from build123d import *

# Parameters (mm, degrees)
SKETCH1_R           = 7.25
BOSS_EXTRUDE1_DEPTH = 3
SKETCH2_R           = 3.5
SKETCH2_R_2         = 2.5
BOSS_EXTRUDE2_DEPTH = 3
SKETCH3_R           = 0.75
CUT_EXTRUDE1_DEPTH  = 12.879604371
CHAMFER1_SIZE       = 0.5
SKETCH5_R           = 1.25
CUT_EXTRUDE3_DEPTH  = 12.879604371


with BuildPart() as part:
    # Sketch1 → Boss-Extrude1 (new body)
    with BuildSketch(Plane.XY):
        Circle(SKETCH1_R)
    extrude(amount=BOSS_EXTRUDE1_DEPTH)

    # Sketch2 → Boss-Extrude2 (add)
    with BuildSketch(Plane(origin=(0, 0, 0), x_dir=(-1, 0, 0), z_dir=(0, 0, -1))):
        with Locations(Location((0, 0, 0), (0, 0, 180))):
            Circle(SKETCH2_R)
        Circle(SKETCH2_R_2, mode=Mode.SUBTRACT)
    extrude(amount=BOSS_EXTRUDE2_DEPTH)

    # Sketch3 → Cut-Extrude1 (cut, through all)
    with BuildSketch(Plane.XY.offset(3)):
        with Locations((0, 5)):
            Circle(SKETCH3_R)
        with Locations((5, 0)):
            Circle(SKETCH3_R)
        with Locations((0, -5)):
            Circle(SKETCH3_R)
        with Locations((-5, 0)):
            Circle(SKETCH3_R)
    extrude(amount=-CUT_EXTRUDE1_DEPTH, mode=Mode.SUBTRACT)

    # Chamfer1
    chamfer1_edges = [part.edges().sort_by_distance(p)[0] for p in [
        (-7.25, 0, 0),
        (-7.25, 0, 3),
        (-3.5, 0, -3),
    ]]
    chamfer(chamfer1_edges, length=CHAMFER1_SIZE)

    # Sketch5 → Cut-Extrude3 (cut, through all)
    with BuildSketch(Plane.XY.offset(3)):
        Circle(SKETCH5_R)
    extrude(amount=-CUT_EXTRUDE3_DEPTH, mode=Mode.SUBTRACT)


solid = part.part
Here's how the part is built. I have some questions about the finished solid (model axes, mm). A direction names the side the tool comes from. Coordinates: 2 decimals unless noted, no trailing zeros. Order: outer loops, then holes, each group sorted by start corner. A loop starts at its lowest first (then second) coordinate and runs counter-clockwise, first axis right, second up. Notation, with made-up numbers: (19.5, 30.25) -> (26.5, 30.25) arc R16 cw to (26.5, 49.25) -> close; hole circle Ø5 at (28, 74.25). An arc over 180 degrees is marked (long way). Answer in a Markdown table with one row per item.
(1) Thinking about a two-plate mould opening in Y: for faces 1 (the face through (3.35, -6.43, 1.49)), 2 (the face through (-0.27, -1.22, 1.52)), 3 (the face through (1.4, 0.1, 3)), 4 (the face through (0.54, -2.44, -1.48)), which applies, +Y half, -Y half, draft (parallel to the pull), parting line (faces both ways), or undercut?
Answer key:
| item | result |
|---|---|
| face 1 | parting line |
| face 2 | undercut |
| face 3 | draft |
| face 4 | undercut |
(2) Will these pins go through, and if not, where does the flat tip stop? pin 1 Ø1 at (x, z) = (-6, 0) entering from -Y; pin 2 Ø4 at (x, y) = (5, -4.5) entering from -Z.
Answer key:
| item | result |
|---|---|
| pin 1 | y = -4.32 |
| pin 2 | z = 0 |
(3) I want a section at A-A on x = 0. Count the separate pieces of the cut face and the enclosed holes in it, then the cut area to 4 significant figures.
Answer key:
| item | result |
|---|---|
| separate pieces | 4 |
| enclosed holes | 0 |
| area | 32.25 mm^2 |
(4) I want a section at C-C on z = 1.45. List the corners of the cut face in (x, y) for me, then the cut area to 3 significant figures.
Answer key:
| item | result |
|---|---|
| outline | circle Ø14.5 at (0, 0); hole circle Ø1.5 at (-5, 0); hole circle Ø2.5 at (0, 0); hole circle Ø1.5 at (0, -5); hole circle Ø1.5 at (0, 5); hole circle Ø1.5 at (5, 0) |
| area | 153 mm^2 |
(5) On a 3-axis mill with a long thin cutter (end or side, diameter ignored), from which of +Z, -Z, +X, -X, +Y, -Y can I reach the whole of each face in a straight line? I mean faces 5 (the face through (3, -3, 0)), 6 (the face through (-2, -2, -3)). Say none if no direction works.
Answer key:
| item | result |
|---|---|
| face 5 | -Z |
| face 6 | -Z, +X, -X, +Y, -Y |
(6) Please list where these lines run through material, in increasing order: probe 1 along Y at (x, z) = (0, 2.3); probe 2 along X at (y, z) = (0.25, 2.6); probe 3 along Z at (x, y) = (-5, -1.25).
Answer key:
| item | result |
|---|---|
| probe 1 | -7.25 to -5.75, -4.25 to -1.25, 1.25 to 4.25, 5.75 to 7.25 |
| probe 2 | -7.15 to -5.71, -4.29 to -1.22, 1.22 to 4.29, 5.71 to 7.15 |
| probe 3 | 0 to 3 |
(7) I want a section at D-D on z = -0.2. List the corners of the cut face in (x, y) for me, then the cut area to 3 significant figures.
Answer key:
| item | result |
|---|---|
| outline | circle Ø7 at (0, 0); hole circle Ø5 at (0, 0) |
| area | 18.8 mm^2 |
